Check sheet for the drawn part. Datum: minimum x, y, z corner. Units: mm. Give positions to 0.01 mm unless a question says otherwise; leave off trailing zeros. Write each loop counter-clockwise with the first axis right and the second up, starting at its lowest first coordinate (ties: lowest second). Pieces come first, ordered by that corner, then holes. Notation, with made-up numbers: (70.25, 3.5) -> (86.25, 3.5) arc R14 cw to (86.25, 17.5) -> close; hole circle Ø7 at (-24.75, 38.5). An arc over 180 degrees is marked (long way). Use CSV: the item, a comma, the result in double quotes. Start each with the question number.
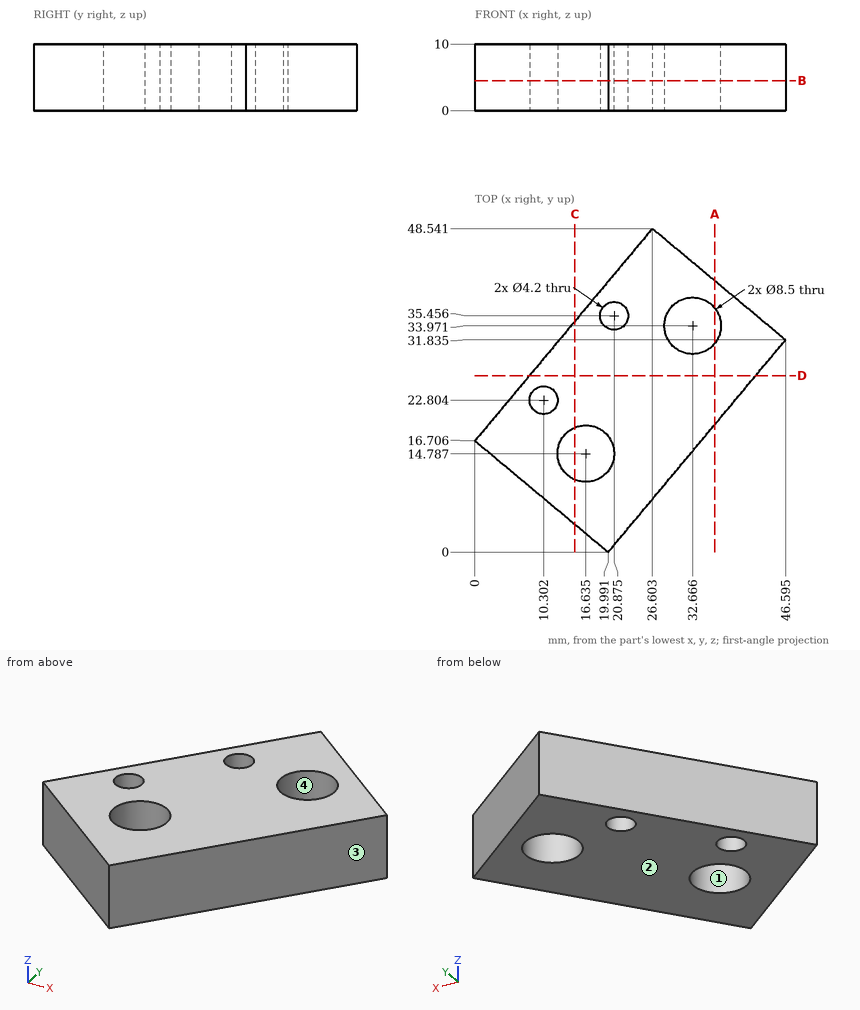
(1) Section check A-A on x = 36. Record the cut outline in (y, z) (1 decimal), then the cut area to 3 significant figures.
(2) Section check C-C on x = 15. Record the cut outline in (y, z).
(3) Section check D-D on y = 26.5. Record the cut outline in (x, z) (1 decimal).
(4) Draft check along Y on the marked faces 1, 2, 3 and 4. Enter one of: released by +Y, released by -Y, zero draft, split by the parting line, or undercut.
(5) Section check B-B on z = 4.5. Give the number of separate pieces and of enclosed holes in the cut face.
(6) Thickness scan on line 1 (X direction, y = 35, z = 6) (1 decimal); line 2 (X direction, y = 35.5, z = 2.5) (1 decimal); line 3 (X direction, y = 21, z = 6.25) (1 decimal). Record the ranges inside material, lowest first. Write a range as from..to.
(7) Go/stop test with flat-tipped pins: pin 1 (7.5 mm diameter, centred on x = 16.63, y = 14.79, fed in from +Z); pin 2 (2 mm diameter, centred on y = 12.5, z = 5, fed in from -X) (1 decimal); pin 3 (2 mm diameter, centred on x = 15, z = 3, fed in from -Y) (1 decimal); pin 4 (4 mm diameter, centred on x = 20.5, z = 6, fed in from -Y). Record where each tip stops, or that it passes through.
Data:
1,outline,"(19.2, 0) -> (31.3, 0) -> (31.3, 10) -> (19.2, 10) -> close; (36.6, 0) -> (40.7, 0) -> (40.7, 10) -> (36.6, 10) -> close"
1,area,"163 mm2"
2,outline,"(4.17, 0) -> (10.86, 0) -> (10.86, 10) -> (4.17, 10) -> close; (18.71, 0) -> (34.66, 0) -> (34.66, 10) -> (18.71, 10) -> close"
3,outline,"(8.2, 0) -> (42.1, 0) -> (42.1, 10) -> (8.2, 10) -> close"
4,face 1,"undercut"
4,face 2,"zero draft"
4,face 3,"released by -Y"
4,face 4,"undercut"
5,separate pieces,"1"
5,enclosed holes,"4"
6,line 1,"x = 15.3..18.8, 22.9..28.5, 36.8..42.8"
6,line 2,"x = 15.7..18.8, 23..28.7, 36.6..42.2"
6,line 3,"x = 3.6..9.2, 11.4..37.5"
7,pin 1,"passes through"
7,pin 2,"stops at x = 3.8"
7,pin 3,"stops at y = 3.3"
7,pin 4,"stops at y = 0"
